Input: dimensioned drawing with shaded views. Units: mm. Origin: part minimum x, y, z. A direction names the side the tool comes from. Give positions to 0.01 mm unless a question says otherwise; leave off trailing zeros. Order: outer loops, then holes, each group sorted by start corner. A loop starts at its lowest first (then second) coordinate and runs counter-clockwise, first axis right, second up. Notation, with made-up numbers: (69, -26) -> (108, -26) arc R27 ccw to (108, 8) -> close; hole circle Ø4 at (30.5, 12.25). An arc over 180 degrees is marked (long way). One line per question, with ' | ' between items. Start each with the question number.
(1) First-contact query: pin 1 Ø3 at (x, y) = (8, 8) entering from +Z. Flat tip, straight axial feed; report the tip coordinate or a pass-through.
(2) Mould query, pull axis X, two halves, no side actions, for the marked faces 3, 4 and 5. Classes: +X half, -X half, draft (parallel to the pull), parting line (faces both ways), or undercut.
(3) Section A-A (x = 7.75). Return loops of the section in (y, z), then the cut area to 3 significant figures.
(4) Ray query, L1, parallel to Y at x = 7.75, z = 1.55; L2, parallel to Y at x = 7.75, z = 0.8; L3, parallel to Z at x = 8, y = 9. Return the intervals inside material, ascending.
(5) Set-up query: the marked faces 1 and 2. Return all of +Z, -Z, +X, -X, +Y, -Y with unobstructed straight access to the full face (end or side cutting, diameter ignored); none if empty.
(6) Section C-C (z = 0.7). Return loops of the section in (x, y), then the cut area to 3 significant figures.
(7) Section D-D (x = 10). Return loops of the section in (y, z), then the cut area to 3 significant figures.
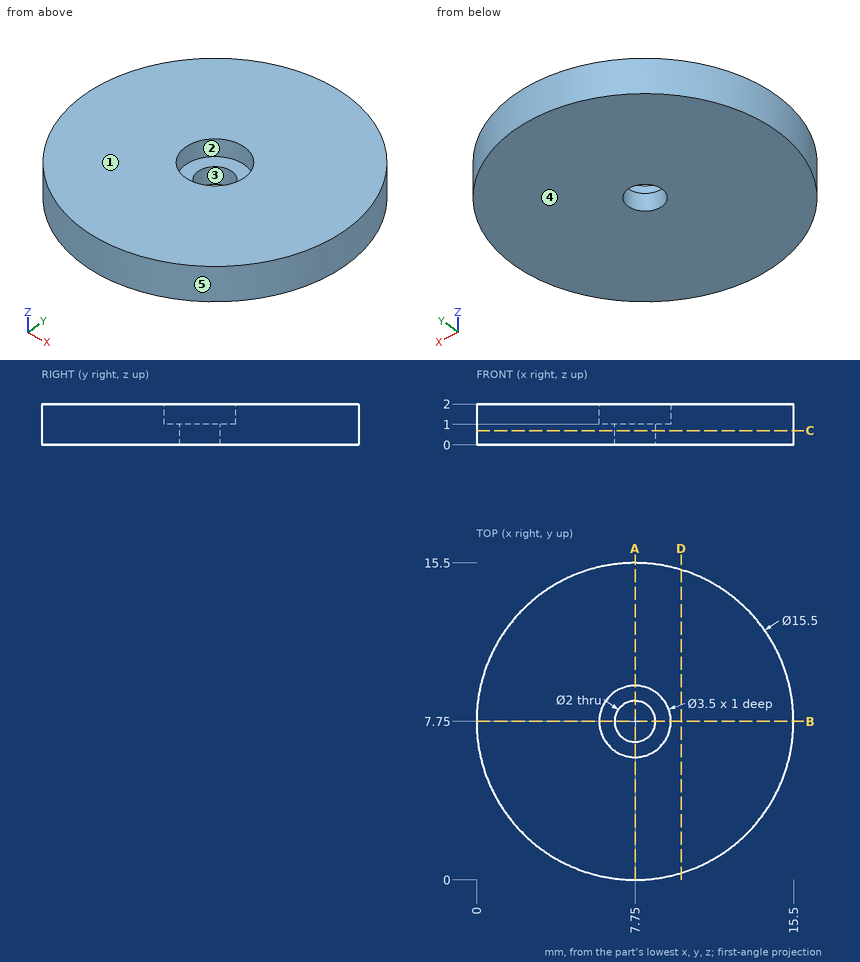
Response:
1) pin 1: stops at z = 2
2) face 3: undercut | face 4: draft | face 5: parting line
3) outline: (0, 0) -> (6.75, 0) -> (6.75, 1) -> (6, 1) -> (6, 2) -> (0, 2) -> close; (8.75, 0) -> (15.5, 0) -> (15.5, 2) -> (9.5, 2) -> (9.5, 1) -> (8.75, 1) -> close | area: 25.5 mm^2
4) L1: y = 0 to 6, 9.5 to 15.5 | L2: y = 0 to 6.75, 8.75 to 15.5 | L3: z = 0 to 1
5) face 1: +Z, +X, -X, +Y, -Y | face 2: +Z
6) outline: circle Ø15.5 at (7.75, 7.75); hole circle Ø2 at (7.75, 7.75) | area: 186 mm^2
7) outline: (0.33, 0) -> (15.17, 0) -> (15.17, 2) -> (0.33, 2) -> close | area: 29.7 mm^2
